Part print with two shaded views. Sizes in mm from the minimum x, y, z corner. Give positions to 0.01 mm unless a question says otherwise; leave off trailing zeros. Write each loop counter-clockwise with the first axis right and the second up, starting at its lowest first coordinate (ties: lowest second). Pieces come first, ordered by that corner, then holes.
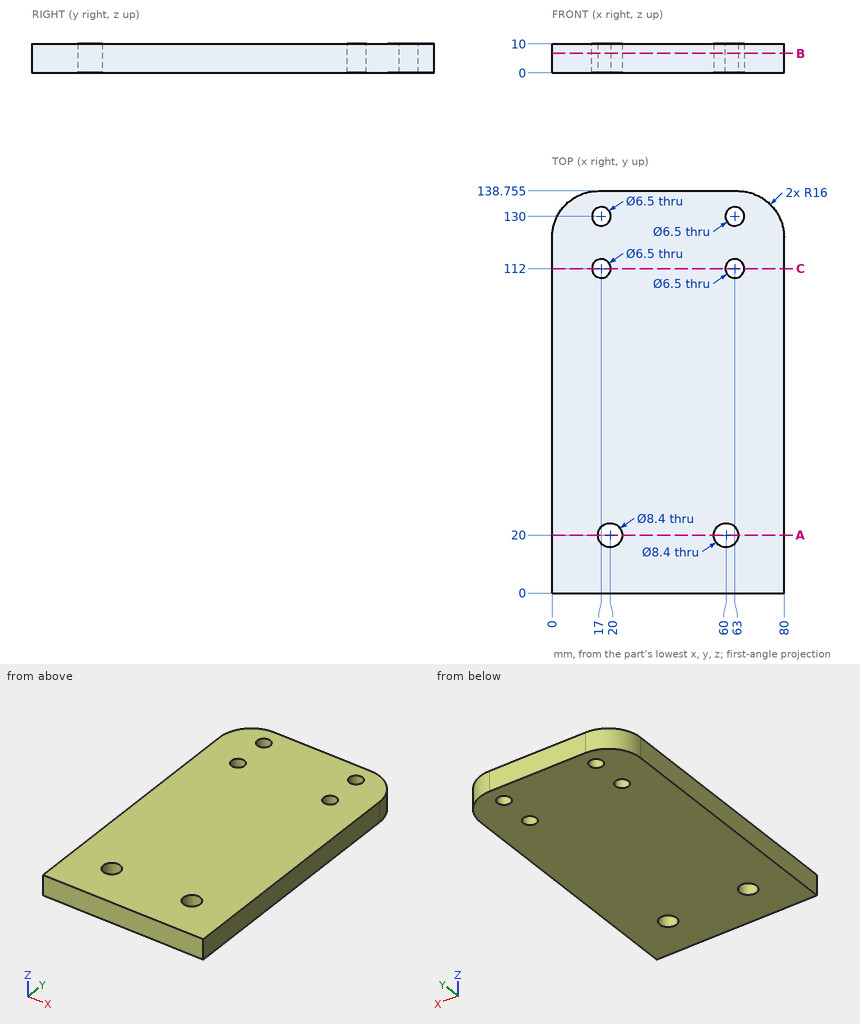
(1) Saw through at A-A, the plane y = 20. List the corners of the cut face in (x, z).
(2) Probe line 1 (Y direction, x = 19, z = 9.25) (1 decimal); line 2 (X direction, y = 123, z = 5.5); line 3 (Y direction, x = 13.5, z = 7). List the from-to ranges inside material, lowest first.
(3) Drop flat-ended pins along their axis: pin 1 (2 mm diameter, centred on y = 124.5, z = 2.5, fed in from -X); pin 2 (5 mm diameter, centred on x = 17, y = 112, fed in from -Z). Give the stop position or say it passes through.
(4) Saw through at C-C, the plane y = 112. List the corners of the cut face in (x, z), plus the area to 3 significant figures.
(5) Saw through at B-B, the plane z = 6.75. Give the number of separate pieces and of enclosed holes in the cut face, plus the area to 3 significant figures.
Computed values:
1. outline: (0, 0) - (15.8, 0) - (15.8, 10) - (0, 10) - close; (24.2, 0) - (55.8, 0) - (55.8, 10) - (24.2, 10) - close; (64.2, 0) - (80, 0) - (80, 10) - (64.2, 10) - close
2. line 1: y = 0 to 15.9, 24.1 to 109.4, 114.6 to 127.4, 132.6 to 138.8
2. line 2: x = 0 to 80
2. line 3: y = 0 to 138.56
3. pin 1: stops at x = 0.02
3. pin 2: passes through
4. outline: (0, 0) - (13.75, 0) - (13.75, 10) - (0, 10) - close; (20.25, 0) - (59.75, 0) - (59.75, 10) - (20.25, 10) - close; (66.25, 0) - (80, 0) - (80, 10) - (66.25, 10) - close
4. area: 670 mm2
5. separate pieces: 1
5. enclosed holes: 6
5. area: 10,700 mm2
